```python
from build123d import *

# Parameters (mm, degrees)
SKETCH1_R           = 14.2748
BOSS_EXTRUDE1_DEPTH = 6.35
SKETCH2_R           = 2.4892
CUT_EXTRUDE1_DEPTH  = 448.798830392
FILLET1_R           = 6.35
SKETCH3_R           = 3.2639
CUT_EXTRUDE2_DEPTH  = 448.798830392
FILLET2_R           = 6.35


with BuildPart() as part:
    # Sketch1 → Boss-Extrude1 (new, symmetric)
    # profile 1 of 2: a face of its own
    with BuildSketch(Plane.XY):
        Polygon((-190.184633538, -88.8238), (-190.184633538, 114.3762), (-304.484633538, 114.3762), (-304.484633538, -88.8238), (-381, -190.5), (-355.6, -190.5), (-355.6, -234.95), (-304.8, -234.95), (-247.334633538, -165.1), (-177.220797536, -165.1), (-177.220797536, -127), (-164.520797536, -127), (-164.520797536, -165.1), (152.979202464, -165.1), (152.979202464, -127), (165.679202464, -127), (165.679202464, -165.1), (191.079202464, -165.1), (191.079202464, -234.95), (229.17754613, -234.95), (229.17754613, -190.5), (251.064839113, -190.5), (251.064839113, -114.2238), (-190.184633538, -114.2238), align=None)
        with Locations((-304.560833538, -136.4488)):
            Circle(SKETCH1_R, mode=Mode.SUBTRACT)
        with Locations((-247.334633538, -136.4488)):
            Circle(SKETCH1_R, mode=Mode.SUBTRACT)
        with Locations((-247.334633538, 79.4512)):
            Circle(SKETCH1_R, mode=Mode.SUBTRACT)
    # profile 2 of 2: a face of its own
    with BuildSketch(Plane.XY):
        Polygon((-190.184633538, -88.8238), (-190.184633538, 114.3762), (-304.484633538, 114.3762), (-304.484633538, -88.8238), (-381, -190.5), (-355.6, -190.5), (-355.6, -234.95), (-304.8, -234.95), (-247.334633538, -165.1), (-177.220797536, -165.1), (-177.220797536, -127), (-164.520797536, -127), (-164.520797536, -165.1), (152.979202464, -165.1), (152.979202464, -127), (165.679202464, -127), (165.679202464, -165.1), (191.079202464, -165.1), (191.079202464, -234.95), (229.17754613, -234.95), (229.17754613, -190.5), (251.064839113, -190.5), (251.064839113, -114.2238), (-190.184633538, -114.2238), align=None)
        with Locations((-304.560833538, -136.4488)):
            Circle(SKETCH1_R, mode=Mode.SUBTRACT)
        with Locations((-247.334633538, -136.4488)):
            Circle(SKETCH1_R, mode=Mode.SUBTRACT)
        with Locations((-247.334633538, 79.4512)):
            Circle(SKETCH1_R, mode=Mode.SUBTRACT)
    extrude(amount=BOSS_EXTRUDE1_DEPTH, both=True)

    # Sketch2 → Cut-Extrude1 (cut, through all)
    with BuildSketch(Plane.XY.offset(6.35)):
        with Locations((-288.22680671, -90.447274763)):
            Circle(SKETCH2_R)
        with Locations((-349.758, -172.212)):
            Circle(SKETCH2_R)
        with Locations((-296.314296632, -192.457816118)):
            Circle(SKETCH2_R)
    extrude(amount=-CUT_EXTRUDE1_DEPTH, mode=Mode.SUBTRACT)

    # Fillet1
    fillet1_edges = [part.edges().sort_by_distance(p)[0] for p in [
        (152.979202464, -127, 0),
        (165.679202464, -127, 0),
        (-164.520797536, -127, 0),
        (-177.220797536, -127, 0),
    ]]
    fillet(fillet1_edges, radius=FILLET1_R - 0.0001)  # a hair under: the kernel refuses the full size

    # Sketch3 → Cut-Extrude2 (cut, through all)
    with BuildSketch(Plane.XY.offset(6.35)):
        with Locations((-189.920797536, -158.75)):
            Circle(SKETCH3_R)
        with Locations((178.379202464, -158.75)):
            Circle(SKETCH3_R)
        with Locations((-151.820797536, -158.75)):
            Circle(SKETCH3_R)
        with Locations((140.279202464, -158.75)):
            Circle(SKETCH3_R)
    extrude(amount=-CUT_EXTRUDE2_DEPTH, mode=Mode.SUBTRACT)

    # Fillet2
    fillet2_edges = [part.edges().sort_by_distance(p)[0] for p in [
        (251.064839113, -190.5, 0),
        (229.17754613, -190.5, 0),
        (229.17754613, -234.95, 0),
        (191.079202464, -234.95, 0),
        (191.079202464, -165.1, 0),
        (165.679202464, -165.1, 0),
        (152.979202464, -165.1, 0),
        (-164.520797536, -165.1, 0),
        (-177.220797536, -165.1, 0),
        (-247.334633538, -165.1, 0),
        (-304.8, -234.95, 0),
        (-355.6, -234.95, 0),
        (-355.6, -190.5, 0),
        (-381, -190.5, 0),
        (-304.484633538, -88.8238, 0),
        (-304.484633538, 114.3762, 0),
        (-190.184633538, 114.3762, 0),
        (-190.184633538, -114.2238, 0),
        (251.064839113, -114.2238, 0),
    ]]
    fillet(fillet2_edges, radius=FILLET2_R)


solid = part.part
```
Model file for the job. Use its own axes, mm. A direction names the side the tool comes from. Round coordinates to 2 decimals unless told otherwise and drop trailing zeros. Write each loop counter-clockwise with the first axis right and the second up, starting at its lowest first coordinate (ties: lowest second). Pieces come first, ordered by that corner, then holes. Notation, with made-up numbers: (46, 78) -> (70, 78) arc R22 ccw to (70, 86) -> close; hole circle Ø2 at (-13, 63). An arc over 180 degrees is marked (long way). Answer as CSV lines item,"result".
1. Slice it at B-B, the plane x = -219.5. List the corners of the cut face in (y, z), plus the area to 3 significant figures.
Resolved:
outline,"(-165.1, -6.35) -> (114.38, -6.35) -> (114.38, 6.35) -> (-165.1, 6.35) -> close"
area,"3,550 mm²"
2. Slice it at C-C, the plane z = 2. State how many separate pieces and enclosed holes the cut face has, plus the area to 3 significant figures.
Resolved:
separate pieces,"1"
enclosed holes,"10"
area,"62,600 mm²"
3. Slice it at D-D, the plane x = -56.5. List the corners of the cut face in (y, z).
Resolved:
outline,"(-165.1, -6.35) -> (-114.22, -6.35) -> (-114.22, 6.35) -> (-165.1, 6.35) -> close"
4. Drill centre lines: line 1 (Y direction, x = 204, z = 4); line 2 (Y direction, x = 186, z = 5.5); line 3 (Y direction, x = -305.5, z = -5.5). Where is each one in solid material? Low to high.
Resolved:
line 1,"-234.95 to -114.22"
line 2,"-165.23 to -114.22"
line 3,"-234.52 to -150.69, -122.2 to -90.15"
5. Pin check, flat tips, straight feed: pin 1 Ø4 at (y, z) = (20, 0.5) entering from -X; pin 2 Ø6.5 at (y, z) = (42.5, -0.5) entering from +X; pin 3 Ø6.5 at (x, z) = (-220, 3) entering from -Y. Stop position of each tip, or through.
Resolved:
pin 1,"x = -304.48"
pin 2,"x = -190.18"
pin 3,"y = -165.1"
6. Slice it at A-A, the plane y = -206.5. List the corners of the cut face in (x, z).
Resolved:
outline,"(-355.6, -6.35) -> (-281.39, -6.35) -> (-281.39, 6.35) -> (-355.6, 6.35) -> close; (191.08, -6.35) -> (229.18, -6.35) -> (229.18, 6.35) -> (191.08, 6.35) -> close"
7. Mould opens along X. For faces 1 (the face through (-234.15, -141.92, -0.09)), 2 (the face through (191.079, -200, 0)), 3 (the face through (210, -234.95, 0)), 4 (the face through (251.065, -153, 0)) say: +X half, -X half, draft (parallel to the pull), parting line (faces both ways), or undercut.
Resolved:
face 1,"undercut"
face 2,"undercut"
face 3,"draft"
face 4,"+X half"
8. Tool access for faces 5 (the face through (-304.485, 12, 0)), 6 (the face through (33, -114.224, 0)), 7 (the face through (-355.6, -213, 0)): list every direction of +Z, -Z, +X, -X, +Y, -Y with a clear straight run to the whole face (end or side of a thin tool).
Resolved:
face 5,"+Z, -Z, -X, +Y"
face 6,"+Z, -Z, +X, +Y"
face 7,"+Z, -Z, -X, -Y"
